Verification items for the finished model (mm, model axes). Face numbers are marked on the shaded views. Give positions to 0.01 mm unless a question says otherwise; leave off trailing zeros. Loops run counter-clockwise (first coordinate to the right, second up) from the corner with the lowest first, then second, coordinate; pieces in that order, holes last. Notation, with made-up numbers: (54, -19) - (84, -19) arc R24 cw to (84, -8) - close; hole circle Ø11 at (-16, 24.25). An arc over 180 degrees is marked (long way). Answer in a Markdown table with one row per item.
Autodesk Inventor part; units mm, degrees
ref_plane "YZ Plane" through (0, 0, 0) normal (1, 0, 0) x (0, 1, 0)
ref_plane "XZ Plane" through (0, 0, 0) normal (0, 1, 0) x (-1, 0, 0)
ref_plane "XY Plane" through (0, 0, 0) normal (0, 0, 1) x (1, 0, 0)
sketch "Sketch1" plane through (0, 0, 0) normal (0, 1, 0) x (-1, 0, 0)
  line L0 (0, 0) -> (0, -21) construction
  line L1 (7, -21) -> (12, -21)
  line L2 (12, -21) -> (12, -19)
  line L3 (12, -19) -> (12.5, -19)
  line L4 (12.5, -19) -> (12.5, -0.5)
  line L5 (12.5, -0.5) -> (12, 0)
  line L6 (12, 0) -> (8.2431, 0)
  line L7 (7, -0.289) -> (7, -21)
  line L8 (8.2431, 0) -> (7.5, 0)
  line L9 (7, -0.289) -> (7.5, 0)
  point P0 (12, -20)
  dimension "d0" = 21
  dimension "d2" = 12
  dimension "d3" = 2
  dimension "d4" = 18.5
  dimension "d5" = 21
  dimension "d6" = 0
  dimension "d7" = 7.5
  dimension "d8" = 0.289
  dimension "d9" = 12.5
  dimension "d10" = 5.5
revolve "Revolution1" add sketch "Sketch1" angle 360 about axis through (0, 0, 0) along (0, 0, -1)
properties part number "26-10-209_ZI01"
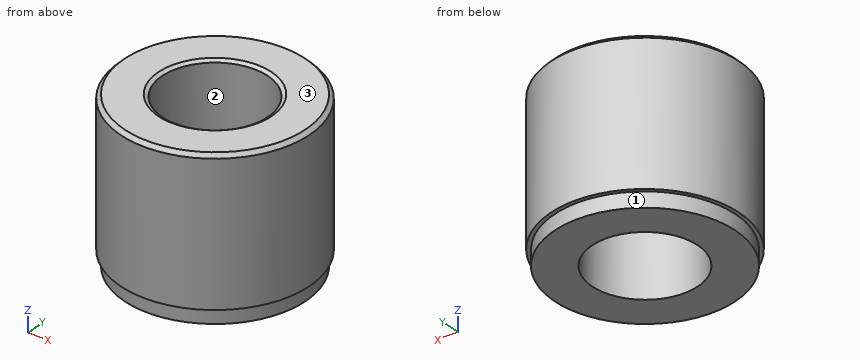
Q1. Sectioned sample at A-A (y = 0). Record the cut outline in (x, z).
Completed:
| item | result |
|---|---|
| outline | (-12.5, -19) - (-12, -19) - (-12, -21) - (-7, -21) - (-7, -0.29) - (-7.5, 0) - (-12, 0) - (-12.5, -0.5) - close; (7, -21) - (12, -21) - (12, -19) - (12.5, -19) - (12.5, -0.5) - (12, 0) - (7.5, 0) - (7, -0.29) - close |
Q2. Draft check along X on the marked faces 1, 2 and 3. Enter one of: +X half, -X half, draft (parallel to the pull), parting line (faces both ways), or undercut.
Completed:
| item | result |
|---|---|
| face 1 | parting line |
| face 2 | undercut |
| face 3 | draft |
Q3. Go/stop test with flat-tipped pins: P1, Ø3, axis at x = 3, z = -3.5, coming from the -Y side; P2, Ø5, axis at y = -9, z = -3.5, coming from the -X side; P3, Ø8, axis at x = -4.5, z = -18, coming from the -Y side. Record where each tip stops, or that it passes through.
Completed:
| item | result |
|---|---|
| P1 | y = -12.41 |
| P2 | x = -10.68 |
| P3 | y = -12.49 |
Q4. Sectioned sample at C-C (z = -12.5). Record the cut outline in (x, y), and give its area (3 significant figures).
Completed:
| item | result |
|---|---|
| outline | circle Ø25 at (0, 0); hole circle Ø14 at (0, 0) |
| area | 337 mm^2 |
Q5. Thickness scan on line 1 (Y direction, x = 0, z = -9); line 2 (X direction, y = 5, z = -12); line 3 (X direction, y = 4.5, z = -7.5). Record the ranges inside material, lowest first.
Completed:
| item | result |
|---|---|
| line 1 | -12.5 to -7, 7 to 12.5 |
| line 2 | -11.46 to -4.9, 4.9 to 11.46 |
| line 3 | -11.66 to -5.36, 5.36 to 11.66 |
